Can you work these out from the model? Positions are in its coordinate system, mm. Coordinates: 2 decimals unless noted, no trailing zeros. Loops run counter-clockwise (first coordinate to the right, second up) from the corner with the lowest first, then second, coordinate; pieces in that order, holes last. Notation, with made-up numbers: M 45.5,59 L 88.5,59 A23 ccw 88.5,77 Z; hole C 78.25,25.5 d9. An arc over 180 degrees is marked long. Answer as a JSON object with one key per item and string values. Group by question number.
Item 1: Suppose I cut it at A-A (y = 1.2). Write out the boundary of the cut face in (x, z) (3 decimals), then the cut area to 3 significant figures.
Item 2: We'd pull the mould along Z, two halves only. Please class faces 1 (the flat face through (1.2, 2.25, 1.2)), 2 (the cylindrical face through (0.45, 1.11, 1.43)), 3 (the flat face through (2.306, 1.109, 1.356)), 4 (the flat face through (2.327, 1.109, -1.319)): +Z half, -Z half, draft (parallel to the pull), parting line (faces both ways), or undercut.
Item 3: I'm going to push a flat-ended pin straight in: pin 1 Ø1 at (y, z) = (2, -1.5) entering from +X. Where does the tip first touch, or does it pass through?
Item 4: If I drill on line 1 (X direction, y = 1.5, z = 1.2); line 2 (Z direction, x = -0.5, y = 2.05) (3 decimals); line 3 (Z direction, x = 0.75, y = 1) (3 decimals), over which ranges is the centre line in solid material (lowest first)?
```python
from build123d import *

# Parameters (mm, degrees)
SKETCH1_R           = 1.5
BOSS_EXTRUDE1_DEPTH = 2.25


with BuildPart() as part:
    # Sketch1 → Boss-Extrude1 (new body)
    with BuildSketch(Plane(origin=(0, 0, 0), x_dir=(1, 0, 0), z_dir=(0, 1, 0))):
        Polygon((1.54441197, 2.675), (-1.54441197, 2.675), (-3.08882394, 0), (-1.54441197, -2.675), (1.54441197, -2.675), (3.08882394, 0), align=None)
        with Locations(Location((0, 0, 0), (0, 0, 270))):
            Circle(SKETCH1_R, mode=Mode.SUBTRACT)
    extrude(amount=BOSS_EXTRUDE1_DEPTH)

    # Sketch2 → Cut-Revolve1 (revolve, cut)
    with BuildSketch(Plane(origin=(0, 0, 0), x_dir=(0, 0, -1), z_dir=(1, 0, 0))):
        with BuildLine():
            Line((0, 2.25), (-2.675, 2.25))
            ThreePointArc((-2.675, 2.25), (-3.012170516, 2.119210025), (-3.17294694, 1.795264171))
            Line((-3.17294694, 1.795264171), (-3.317266919, 1.795264171))
            Line((-3.317266919, 1.795264171), (-3.317266919, 2.57459206))
            Line((-3.317266919, 2.57459206), (0, 2.57459206))
            Line((0, 2.57459206), (0, 2.25))
        make_face()
        with BuildLine():
            Line((0, -0.32459206), (0, 0))
            Line((0, 0), (-2.675, 0))
            ThreePointArc((-2.675, 0), (-3.012170516, 0.130789975), (-3.17294694, 0.454735829))
            Line((-3.17294694, 0.454735829), (-3.317266919, 0.454735829))
            Line((-3.317266919, 0.454735829), (-3.317266919, -0.32459206))
            Line((-3.317266919, -0.32459206), (0, -0.32459206))
        make_face()
    revolve(axis=Axis((0, 2.25, 0), (0, -1, 0)), mode=Mode.SUBTRACT)


solid = part.part
```
From the geometry:
{
 "1": {"outline": "M -3.089,0 L -1.544,-2.675 L 1.544,-2.675 L 3.089,0 L 1.544,2.675 L -1.544,2.675 Z; hole C 0,0 d3", "area": "17.7 mm2"},
 "2": {"face 1": "draft", "face 2": "undercut", "face 3": "+Z half", "face 4": "-Z half"},
 "3": {"pin 1": "x = 2.51"},
 "4": {"line 1": "-2.4 to -0.9, 0.9 to 2.4", "line 2": "-2.675 to -1.414, 1.414 to 2.675", "line 3": "-2.675 to -1.299, 1.299 to 2.675"}
}
